For this review, use the dimensioned drawing (mm, ordinates from the lowest corner) and the shaded views. A direction names the side the tool comes from. Round coordinates to 2 decimals unless told otherwise and drop trailing zeros. Write each loop counter-clockwise with the first axis right and the second up, starting at its lowest first coordinate (ties: lowest second). Pieces come first, ordered by that corner, then holes. Notation, with made-up numbers: M 14,-8.5 L 43,-8.5 A28 cw 43,16.5 Z; hole C 88.5,64.25 d11. An arc over 180 degrees is marked long. Answer in a Markdown table with one row per item.
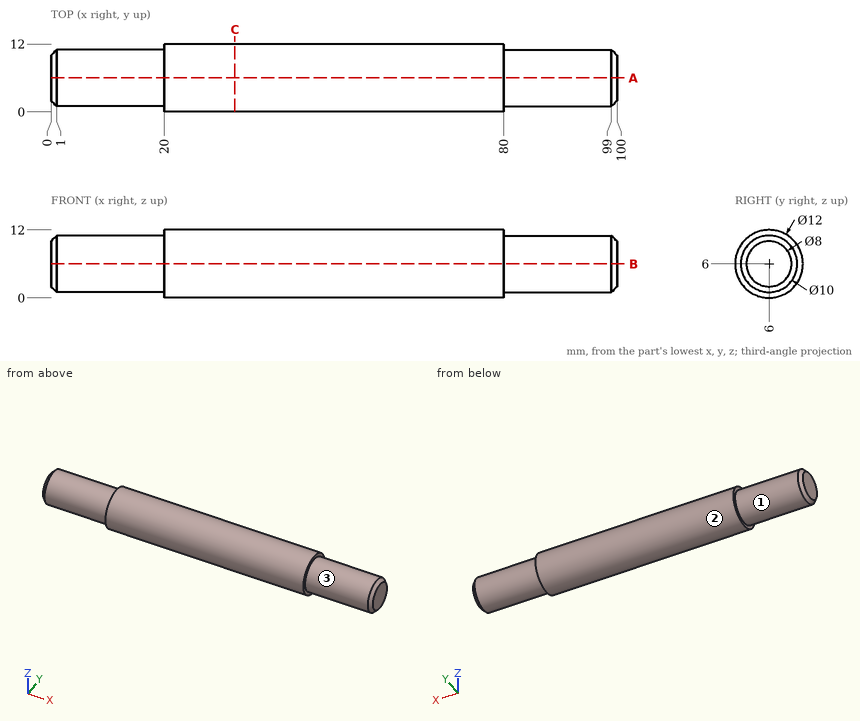
Q1. For probe 1 along X at (y, z) = (1.25, 3.5); probe 2 along Y at (x, z) = (84, 9); probe 3 along Z at (x, y) = (5.5, 6), list the stretches that pass through material, from the lowest coordinate up.
Found:
| item | result |
|---|---|
| probe 1 | 20 to 80 |
| probe 2 | 2 to 10 |
| probe 3 | 1 to 11 |
Q2. Machinability: for the marked faces 1, 2 and 3, which of the approach directions +Z, -Z, +X, -X, +Y, -Y give a long, thin tool a straight path to every point of the face, cutting with its end or side? Answer none if there is none.
Found:
| item | result |
|---|---|
| face 1 | -X |
| face 2 | +X, -X |
| face 3 | +X |
Q3. Take a section at A-A (y = 6). State the section outline as (x, z) points, then the cut area to 3 significant figures.
Found:
| item | result |
|---|---|
| outline | M 0,2 L 1,1 L 20,1 L 20,0 L 80,0 L 80,1 L 99,1 L 100,2 L 100,10 L 99,11 L 80,11 L 80,12 L 20,12 L 20,11 L 1,11 L 0,10 Z |
| area | 1,120 mm² |
Q4. Insertion check: P1, Ø1, axis at x = 26, y = 1.5, coming from the +Z side. The pin has a flat end and moves straight along its axis. Give the tip position at first contact, or say it passes through.
Found:
| item | result |
|---|---|
| P1 | z = 10.47 |
Q5. Take a section at C-C (x = 32.5). State the section outline as (y, z) points, then the cut area to 3 significant figures.
Found:
| item | result |
|---|---|
| outline | C 6,6 d12 |
| area | 113 mm² |
